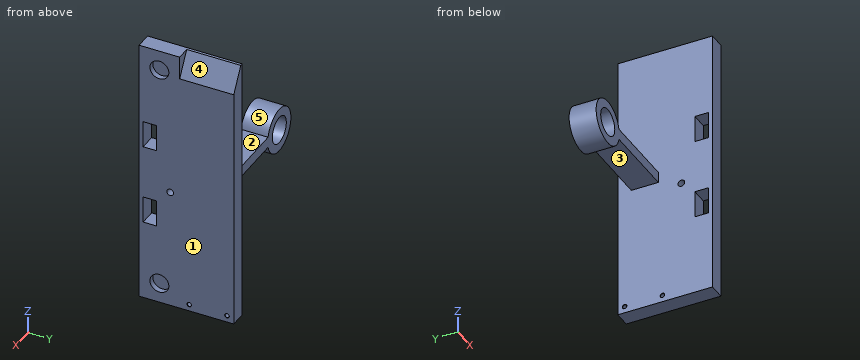
Autodesk Inventor part; units mm, degrees
ref_plane "YZ Plane" through (0, 0, 0) normal (1, 0, 0) x (0, 1, 0)
ref_plane "XZ Plane" through (0, 0, 0) normal (0, 1, 0) x (-1, 0, 0)
ref_plane "XY Plane" through (0, 0, 0) normal (0, 0, 1) x (1, 0, 0)
sketch "Эскиз1" plane through (0, 0, 0) normal (1, 0, 0) x (0, 1, 0)
  line L0 (0, 100) -> (0, -100)
  line L1 (0, -100) -> (30, -100)
  line L2 (30, -100) -> (30, 100)
  line L3 (30, 100) -> (0, 100)
  line L4 (-14, 0) -> (84, 0) construction
  line L5 (0, -140) -> (0, 140) construction
  line L6 (30, -100) -> (70, -100)
  line L7 (70, -100) -> (70, 100)
  line L8 (70, 100) -> (30, 100)
  line L9 (30, 100) -> (30, -100)
  point P0 (0, 0)
  point P1 (30, 100)
  dimension "d0" = 200
  dimension "d1" = 30
  dimension "d2" = 200
  dimension "d3" = 40
extrude "Выдавливание1" add sketch "Эскиз1" along normal mid plane 12
sketch "Эскиз2" plane through (6, 0, 0) normal (1, 0, 0) x (0, 0, -1)
  line L0 (-20, 13) -> (-40, 13)
  line L1 (-100, 0) -> (100, 0) construction
  line L2 (100, 0) -> (100, 70)
  line L3 (-40, 13) -> (-20, 13)
  line L4 (-20, 13) -> (-20, 3)
  line L5 (-20, 3) -> (-40, 3)
  line L6 (-40, 3) -> (-40, 13)
  line L7 (20, 13) -> (40, 13)
  line L8 (40, 13) -> (40, 3)
  line L9 (40, 3) -> (20, 3)
  line L10 (20, 3) -> (20, 13)
  point P0 (0, 0)
  point P1 (-85, 0)
  point P2 (57.0517, 0.6179)
  dimension "d26" = 10
  dimension "d27" = 20
  dimension "d28" = 3
  dimension "d29" = 20
  dimension "d31" = 20
  dimension "d34" = 3
  dimension "d35" = 10
  dimension "d36" = 20
extrude "Выдавливание2" cut sketch "Эскиз2" against normal blind 12
sketch "Эскиз3" plane through (6, 0, 0) normal (1, 0, 0) x (0, 0, -1)
  line L0 (100, 0) -> (100, 70)
  line L1 (100, 0) -> (-100, 0)
  line L2 (-100, 0) -> (-100, 70)
  point P0 (0, 0)
  point P1 (-85, 15)
  point P2 (-85, 0)
  point P3 (-85, 15)
  point P4 (85, 15)
  point P5 (-100, 15)
  dimension "d17" = 15
  dimension "d53" = 15
  dimension "d54" = 15
hole "Отверстие1" at (6, 15, -85) at (6, 15, 85) direction (-1, 0, 0) diameter 14 depth 4.1
sketch "Эскиз4" plane through (6, 0, 0) normal (1, 0, 0) x (0, 0, -1)
  line L0 (100, 70) -> (-100, 70)
  line L1 (-100, 70) -> (-100, 0)
  line L2 (90, 30) -> (-85, 30)
  line L3 (100, 0) -> (100, 70)
  line L4 (100, 0) -> (-100, 0)
  point P0 (0, 0)
  point P1 (95, 65)
  point P2 (95, 37)
  point P3 (-100, 15)
  point P4 (-85, 0)
  dimension "d37" = 5
  dimension "d40" = 5
  dimension "d51" = 5
  dimension "d52" = 37
hole "Отверстие2" at (6, 65, -95) at (6, 37, -95) direction (-1, 0, 0) diameter 3 depth 70
chamfer "Фаска1" distance 0.2 angle 45 4 edges at (6, 37, -93.5) (6, 65, -93.5) (-6, 37, -93.5) (-6, 65, -93.5)
sketch "Эскиз5" plane through (-6, 70, 100) normal (0, 1, 0) x (1, 0, 0)
  line L0 (12, 0) -> (0, 0)
  line L1 (2, 0) -> (12, 17.3205)
  line L2 (12, 200) -> (12, 0)
  line L3 (12, 0) -> (2, 0)
  line L4 (12, 15) -> (12, 0)
  line L5 (12, 0) -> (12, 17.3205)
  point P0 (6, 100)
  dimension "d60" = 30
  dimension "d61" = 10
extrude "Выдавливание3" cut sketch "Эскиз5" against normal blind 40
sketch "Эскиз6" plane through (-6, 0, 0) normal (-1, 0, 0) x (0, 0, 1)
  line L0 (-40, 13) -> (-20, 13)
  point P0 (0, 0)
  point P1 (-10, 23)
  dimension "d62" = 10
  dimension "d63" = 10
hole "Отверстие3" at (-6, 23, -10) direction (1, 0, 0) diameter 5 depth 60
sketch "Эскиз7" plane through (-6, 0, 0) normal (-1, 0, 0) x (0, 0, 1)
  line L0 (-4, 60) -> (4, 60)
  line L1 (4, 60) -> (4, 40)
  line L2 (4, 40) -> (-4, 40)
  line L3 (-4, 40) -> (-4, 60)
  line L4 (0, 0) -> (0, 6.9143) construction
  line L5 (-100, 0) -> (100, 0)
  dimension "d71" = 8
  dimension "d72" = 20
  dimension "d73" = 40
extrude "Выдавливание4" add sketch "Эскиз7" along normal blind 61
sketch "Эскиз10" plane through (-6, 40, -4) normal (0, -1, 0) x (1, 0, 0)
  line L0 (-104, -147.0883) -> (-50, -147.0883)
  line L1 (-50, 252.9117) -> (-50, -147.0883) construction
  circle A0 centre (-72.15, -8.6973) radius 16.5 construction
  circle A1 centre (-72.15, -8.6973) radius 10 construction
  circle A2 centre (-72.15, -8.6973) radius 10 construction
  circle A3 centre (-72.15, -8.6973) radius 11 construction
  circle A4 centre (-72.15, 4) radius 16.5
  circle A5 centre (-72.15, 4) radius 11
  circle A6 centre (-72.15, 4) radius 10
  line L2 (-50, 252.9117) -> (-104, 252.9117)
  line L3 (-104, -147.0883) -> (-104, 252.9117)
  point P0 (6, 4)
  point P1 (-100, 252.9117)
  dimension "d86" = 33
  dimension "d87" = 22
  dimension "d88" = 20
extrude "Выдавливание6" add sketch "Эскиз10" against normal blind 20 contours A4 | A5
properties part number "Стенка конвейера"
Design review of the part built by this model. Coordinates are the model's own, in mm. Face numbers are marked on the shaded views. A direction names the side the tool comes from. Coordinates: 2 decimals unless noted, no trailing zeros. Order: outer loops, then holes, each group sorted by start corner. A loop starts at its lowest first (then second) coordinate and runs counter-clockwise, first axis right, second up. Notation, with made-up numbers: (40, -10.75) -> (55, -10.75) arc R14 ccw to (55, -6.75) -> close; hole circle Ø2 at (65, -16.75). An arc over 180 degrees is marked (long way). One line per item, written item: value. Start each with the question number.
Q1. For probe 1 along Z at (x, y) = (5, 15); probe 2 along Y at (x, z) = (-2.25, -95); probe 3 along Z at (x, y) = (1.5, 23), list the stretches that pass through material, from the lowest coordinate up.
Q2. Take a section at B-B, the plane z = -22.5. State the section outline as (x, y) points.
Q3. Insertion check: pin 1 Ø3.5 at (y, z) = (65, -95) entering from -X; pin 2 Ø16 at (x, y) = (-47, 48.5) entering from -Z; pin 3 Ø4 at (y, z) = (18, -85.5) entering from +X; pin 4 Ø15.5 at (y, z) = (18, 85) entering from +X. Each pin has a flat end and moves straight along its axis. Give the tip position at first contact, or say it passes through.
Q4. Mouldability with a two-part tool opening along X and no side actions: class the marked faces 4 and 5 as pulls with the +X half, pulls with the -X half, needs draft (parallel to the pull), parting line crosses it, or undercut.
Q5. Take a section at D-D, the plane z = -85. State the section outline as (x, y) points, then the cut area to 3 significant figures.
Q6. Take a section at C-C, the plane y = 51.5. State the section outline as (x, z) points.
Q7. Take a section at A-A, the plane x = -78.15. State the section outline as (y, z) points.
Q8. Tool access review of the marked faces 1, 2 and 3: name each direction out of +Z, -Z, +X, -X, +Y, -Y from which nothing blocks a thin tool from reaching the whole face with its end or side.
Values follow:
1. probe 1: z = -100 to -92, -78 to 78, 92 to 100
1. probe 2: y = 0 to 35.5, 38.5 to 63.5, 66.5 to 70
1. probe 3: z = -100 to -12.5, -7.5 to 100
2. outline: (-6, 0) -> (6, 0) -> (6, 3) -> (-6, 3) -> close; (-6, 13) -> (6, 13) -> (6, 70) -> (-6, 70) -> close
3. pin 1: stops at x = -6
3. pin 2: stops at z = -4
3. pin 3: stops at x = 1.9
3. pin 4: stops at x = 6
4. face 4: pulls with the +X half
4. face 5: undercut
5. outline: (-6, 0) -> (6, 0) -> (6, 8) -> (1.9, 8) -> (1.9, 22) -> (6, 22) -> (6, 70) -> (-6, 70) -> close
5. area: 783 mm2
6. outline: (-62.14, -4) -> (-6, -4) -> (-6, -100) -> (6, -100) -> (6, 82.68) -> (-4, 100) -> (-6, 100) -> (-6, 4) -> (-62.14, 4) arc R16.5 ccw (long way) to start; hole circle Ø20 at (-78.15, 0)
7. outline: (40, -16.5) -> (60, -16.5) -> (60, -10) -> (40, -10) -> close; (40, 10) -> (60, 10) -> (60, 16.5) -> (40, 16.5) -> close
8. face 1: +Z, -Z, +X, +Y, -Y
8. face 2: +Z, +Y, -Y
8. face 3: -Z, +Y, -Y
